Geometry: final body of the model. Coordinates: model frame, mm. Face numbers are marked on the shaded views. A direction names the side the tool comes from. Round coordinates to 2 decimals unless told otherwise and drop trailing zeros. Loops run counter-clockwise (first coordinate to the right, second up) from the corner with the lowest first, then second, coordinate; pieces in that order, holes last. Notation, with made-up numbers: M 5.5,-36 L 27.5,-36 A18 cw 27.5,-1 Z; hole C -40,-6.75 d10. An arc over 180 degrees is marked long. Answer as a JSON object with one key per item and string values.
from build123d import *

# Parameters (mm, degrees)
BOSS_EXTRUDE1_DEPTH = 152.4


with BuildPart() as part:
    # Sketch1 → Boss-Extrude1 (new body)
    with BuildSketch(Plane(origin=(0, 0, 0), x_dir=(1, 0, 0), z_dir=(0, 1, 0))):
        with BuildLine():
            ThreePointArc((3.175, 12.296722124), (0, 12.7), (-3.175, 12.296722124))
            Line((-3.175, 12.296722124), (3.175, 12.296722124))
        make_face()
        with BuildLine():
            Line((3.175, 12.296722124), (-3.175, 12.296722124))
            ThreePointArc((-3.175, 12.296722124), (-8.980256121, 8.980256121), (-12.296722124, 3.175))
            ThreePointArc((-12.296722124, 3.175), (-12.7, 0), (-12.296722124, -3.175))
            ThreePointArc((-12.296722124, -3.175), (-8.980256121, -8.980256121), (-3.175, -12.296722124))
            ThreePointArc((-3.175, -12.296722124), (0, -12.7), (3.175, -12.296722124))
            ThreePointArc((3.175, -12.296722124), (8.980256121, -8.980256121), (12.296722124, -3.175))
            ThreePointArc((12.296722124, -3.175), (12.598777143, -1.600254515), (12.7, 0))
            ThreePointArc((12.7, 0), (12.598777143, 1.600254515), (12.296722124, 3.175))
            ThreePointArc((12.296722124, 3.175), (8.980256121, 8.980256121), (3.175, 12.296722124))
        make_face()
        with BuildLine():
            ThreePointArc((-12.296722124, -3.175), (-12.7, 0), (-12.296722124, 3.175))
            Line((-12.296722124, 3.175), (-24.996722124, 3.175))
            Line((-24.996722124, 3.175), (-24.996722124, -3.175))
            Line((-24.996722124, -3.175), (-12.296722124, -3.175))
        make_face()
        with BuildLine():
            ThreePointArc((3.175, -12.296722124), (0, -12.7), (-3.175, -12.296722124))
            Line((-3.175, -12.296722124), (-3.175, -24.996722124))
            Line((-3.175, -24.996722124), (3.175, -24.996722124))
            Line((3.175, -24.996722124), (3.175, -12.296722124))
        make_face()
        with BuildLine():
            Line((24.996722124, 3.175), (12.296722124, 3.175))
            ThreePointArc((12.296722124, 3.175), (12.598777143, 1.600254515), (12.7, 0))
            ThreePointArc((12.7, 0), (12.598777143, -1.600254515), (12.296722124, -3.175))
            Line((12.296722124, -3.175), (24.996722124, -3.175))
            Line((24.996722124, -3.175), (24.996722124, 3.175))
        make_face()
        with BuildLine():
            Line((-3.175, 24.996722124), (-3.175, 12.296722124))
            ThreePointArc((-3.175, 12.296722124), (0, 12.7), (3.175, 12.296722124))
            Line((3.175, 12.296722124), (3.175, 24.996722124))
            Line((3.175, 24.996722124), (-3.175, 24.996722124))
        make_face()
    extrude(amount=BOSS_EXTRUDE1_DEPTH)


solid = part.part
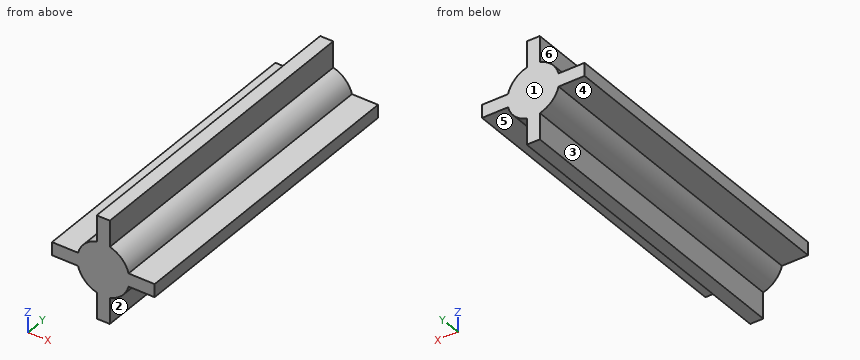
1) Pull-direction query (X, two-part tool) for the marked faces 1, 2 and 3; classes: +X half, -X half, draft (parallel to the pull), parting line (faces both ways), or undercut.
Results:
{"face 1": "draft", "face 2": "+X half", "face 3": "-X half"}
2) Section query B-B (z = -19). Return the cut outline in (x, y) (3 decimals), and give its area (3 significant figures).
Results:
{"outline": "M -3.175,0 L 3.175,0 L 3.175,152.4 L -3.175,152.4 Z", "area": "968 mm2"}
3) Pin query (flat end, axial travel): P1, Ø14, axis at x = 20.5, y = 82.5, coming from the -Z side (3 decimals); P2, Ø4, axis at x = -20, y = 44.5, coming from the +Z side (3 decimals); P3, Ø10, axis at y = 28, z = -18.5, coming from the +X side (3 decimals). Return the tip coordinate at first contact, or that it passes through.
Results:
{"P1": "z = -3.175", "P2": "z = 3.175", "P3": "x = 3.175"}
4) Section query C-C (x = -7). Return the cut outline in (y, z).
Results:
{"outline": "M 0,-10.6 L 152.4,-10.6 L 152.4,10.6 L 0,10.6 Z"}
5) Section query A-A (y = 16). Return the cut outline in (x, z) (3 decimals), and give its area (3 significant figures).
Results:
{"outline": "M -24.997,-3.175 L -12.297,-3.175 A12.7 ccw -3.175,-12.297 L -3.175,-24.997 L 3.175,-24.997 L 3.175,-12.297 A12.7 ccw 12.297,-3.175 L 24.997,-3.175 L 24.997,3.175 L 12.297,3.175 A12.7 ccw 3.175,12.297 L 3.175,24.997 L -3.175,24.997 L -3.175,12.297 A12.7 ccw -12.297,3.175 L -24.997,3.175 Z", "area": "822 mm2"}
6) Reachability of the marked faces 4, 5 and 6 from +Z, -Z, +X, -X, +Y, -Y: full face, straight path, thin tool, end or side. Return the list, or none.
Results:
{"face 4": "-Z, -X, +Y, -Y", "face 5": "-Z, +X, +Y, -Y", "face 6": "+Z, -X, +Y, -Y"}
7) Ray query, line 1 (X direction, y = 139.5, z = -16) (3 decimals); line 2 (X direction, y = 144, z = 3.5). Return the intervals inside material, ascending.
Results:
{"line 1": "-3.175 to 3.175", "line 2": "-12.21 to 12.21"}
